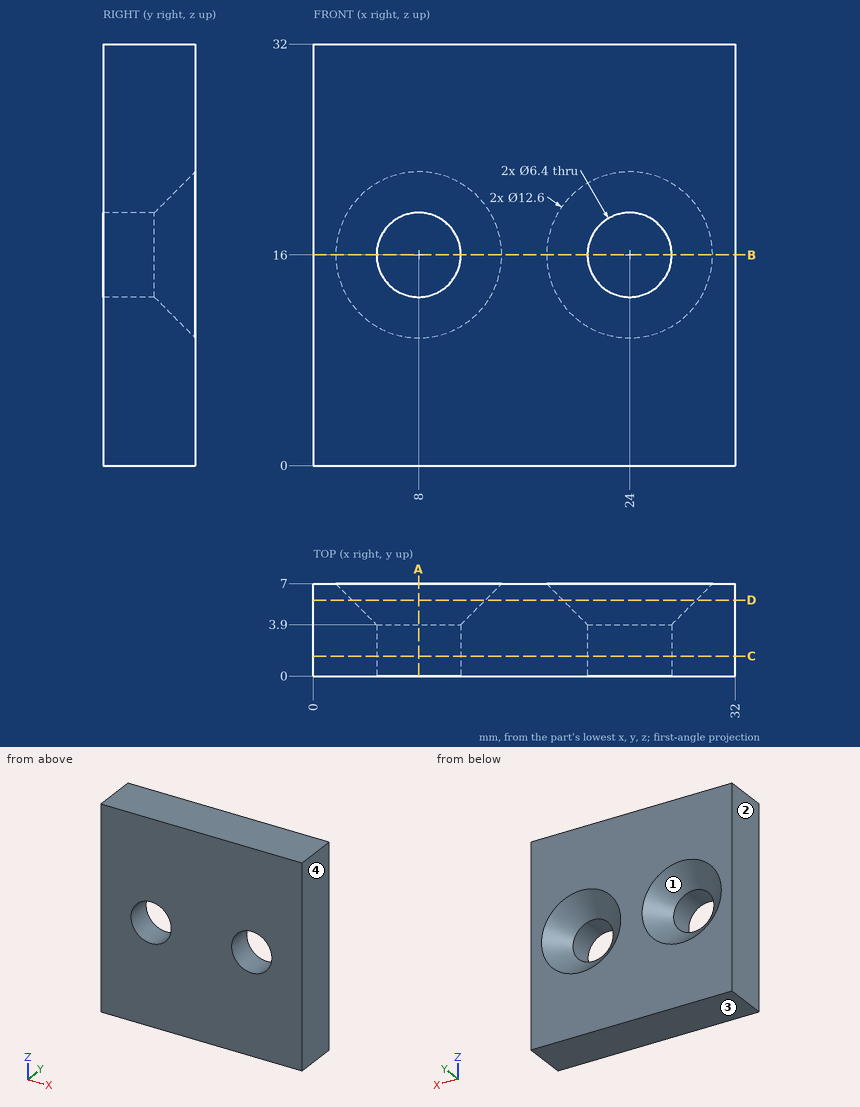
Study the drawing (mm; zero at the part's minimum x, y, z) and answer. Give positions to 0.01 mm unless a question says otherwise; leave off trailing zeros. Write each loop counter-clockwise with the first axis right and the second up, starting at its lowest first coordinate (ties: lowest second). Pieces come first, ordered by that corner, then holes.
(1) The mould has two halves that part along X. Classify the marked faces 1, 2, 3 and 4: pulls with the +X half, pulls with the -X half, needs draft (parallel to the pull), parting line crosses it, or undercut.
Final values:
face 1: undercut
face 2: pulls with the -X half
face 3: needs draft
face 4: pulls with the +X half
(2) The part is cut by section C-C on y = 1.5. Write down the section's boundary in (x, z).
Final values:
outline: (0, 0) - (32, 0) - (32, 32) - (0, 32) - close; hole circle Ø6.4 at (8, 16); hole circle Ø6.4 at (24, 16)
(3) The part is cut by section D-D on y = 5.75. Write down the section's boundary in (x, z).
Final values:
outline: (0, 0) - (32, 0) - (32, 32) - (0, 32) - close; hole circle Ø10.1 at (8, 16); hole circle Ø10.1 at (24, 16)
(4) A flat-ended cylindrical pin translates along its axis: pin 1 Ø5 at (x, z) = (8, 16) entering from +Y. Find the tip coordinate at first contact, or state that the pin passes through.
Final values:
pin 1: passes through
(5) The part is cut by section B-B on z = 16. Write down the section's boundary in (x, y), plus the area to 3 significant figures.
Final values:
outline: (0, 0) - (4.8, 0) - (4.8, 3.9) - (1.7, 7) - (0, 7) - close; (11.2, 0) - (20.8, 0) - (20.8, 3.9) - (17.7, 7) - (14.3, 7) - (11.2, 3.9) - close; (27.2, 0) - (32, 0) - (32, 7) - (30.3, 7) - (27.2, 3.9) - close
area: 115 mm2
(6) The part is cut by section A-A on x = 8. Write down the section's boundary in (y, z).
Final values:
outline: (0, 0) - (7, 0) - (7, 9.7) - (3.9, 12.8) - (0, 12.8) - close; (0, 19.2) - (3.9, 19.2) - (7, 22.3) - (7, 32) - (0, 32) - close
(7) Straight lines are drawn through the part: line 1 (X direction, y = 3.15, z = 16); line 2 (Z direction, x = 24, y = 3.15); line 3 (X direction, y = 4.25, z = 13). For each, find the intervals that lie inside material, in ascending order.
Final values:
line 1: x = 0 to 4.8, 11.2 to 20.8, 27.2 to 32
line 2: z = 0 to 12.8, 19.2 to 32
line 3: x = 0 to 6.1, 9.9 to 22.1, 25.9 to 32
